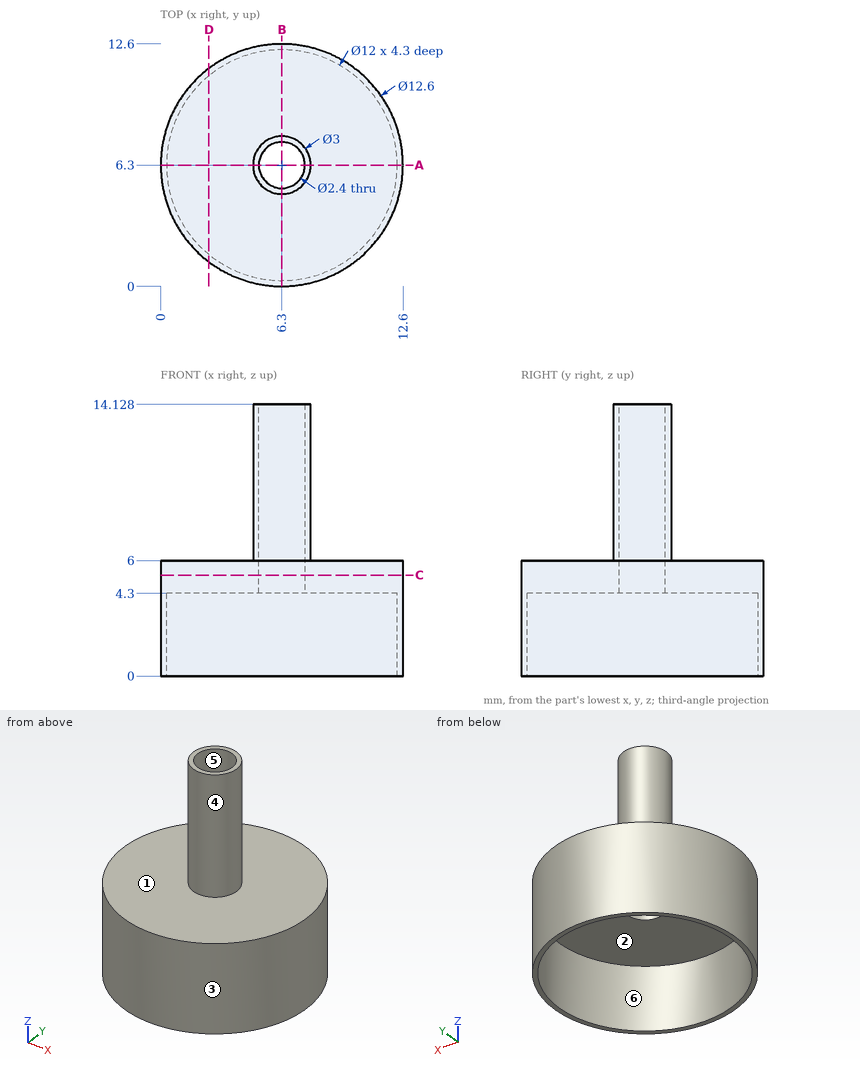
Input: dimensioned drawing with shaded views. Units: mm. Origin: part minimum x, y, z. A direction names the side the tool comes from. Coordinates: 2 decimals unless noted, no trailing zeros. Order: outer loops, then holes, each group sorted by start corner. A loop starts at its lowest first (then second) coordinate and runs counter-clockwise, first axis right, second up.
(1) Material intervals for probe 1 along Y at (x, z) = (6.3, 9.75); probe 2 along Y at (x, z) = (6.3, 1.5); probe 3 along Z at (x, y) = (7.25, 5.25), sorted ascending.
(2) Section query D-D (x = 2.5). Return the cut outline in (y, z).
(3) Section query A-A (y = 6.3). Return the cut outline in (x, z), plus the area to 3 significant figures.
(4) Draft query along X for the marked faces 1, 2 and 3. Return one class per face: pulls with the +X half, pulls with the -X half, needs draft (parallel to the pull), parting line crosses it, or undercut.
(5) Access query for the marked faces 4, 5 and 6. Directions: +Z, -Z, +X, -X, +Y, -Y. A direction counts if a zero-diameter tool reaches every point of the face in a straight line with its end or side. Return the directions, or none.
(6) Section query C-C (z = 5.25). Return the cut outline in (x, y), plus the area to 3 significant figures.
(7) First-contact query: pin 1 (2 mm diameter, centred on x = 9.5, y = 7, fed in from +Z); pin 2 (4 mm diameter, centred on y = 9, z = 12.5, fed in from -X); pin 3 (3 mm diameter, centred on x = 10.5, z = 2, fed in from -Y); pin 4 (1.9 mm diameter, centred on x = 6.3, y = 6.3, fed in from +Z). Flat tips, straight axial feed; report the tip coordinate or a pass-through.
Solution:
1. probe 1: y = 4.8 to 5.1, 7.5 to 7.8
1. probe 2: y = 0 to 0.3, 12.3 to 12.6
1. probe 3: z = 4.3 to 14.13
2. outline: (1.28, 0) - (1.66, 0) - (1.66, 4.3) - (10.94, 4.3) - (10.94, 0) - (11.32, 0) - (11.32, 6) - (1.28, 6) - close
3. outline: (0, 0) - (0.3, 0) - (0.3, 4.3) - (5.1, 4.3) - (5.1, 14.13) - (4.8, 14.13) - (4.8, 6) - (0, 6) - close; (7.5, 4.3) - (12.3, 4.3) - (12.3, 0) - (12.6, 0) - (12.6, 6) - (7.8, 6) - (7.8, 14.13) - (7.5, 14.13) - close
3. area: 24.8 mm2
4. face 1: needs draft
4. face 2: undercut
4. face 3: parting line crosses it
5. face 4: +Z
5. face 5: +Z, -Z
5. face 6: -Z
6. outline: circle Ø12.6 at (6.3, 6.3); hole circle Ø2.4 at (6.3, 6.3)
6. area: 120 mm2
7. pin 1: stops at z = 6
7. pin 2: stops at x = 4.97
7. pin 3: stops at y = 0.61
7. pin 4: passes through
